```python
from build123d import *

# Parameters (mm, degrees)
F0_W     = 190
F0_H     = 100
F1_DEPTH = 30
F2_T     = -5
F4_DEPTH = 100
F5_R     = 3


with BuildPart() as f1:
    # F0 (on Top) → F1 (new body)
    with BuildSketch(Plane.XY):
        Rectangle(F0_W, F0_H)
    extrude(amount=F1_DEPTH)

    # F2
    f2_openings = [f1.faces().sort_by_distance(p)[0] for p in [
        (0, 0, 30),
    ]]
    offset(amount=F2_T, openings=f2_openings)

    # F3 (on face) → F4 (cut, through all)
    with BuildSketch(Plane.XZ.offset(50)):
        with BuildLine():
            ThreePointArc((-5.1e-08, 5), (8.8388347468, 8.6611652172), (12.5, 17.5))
            Line((12.5, 17.5), (-12.5, 17.5))
            ThreePointArc((-12.5, 17.5), (-8.8388347828, 8.6611652532), (-5.1e-08, 5))
        make_face()
        with BuildLine():
            ThreePointArc((-12.5, 17.5), (-8.8388347699, 26.3388347597), (-1.44e-08, 30))
            Line((-1.44e-08, 30), (-12.5, 30))
            Line((-12.5, 30), (-12.5, 17.5))
        make_face()
        with BuildLine():
            Line((-12.5, 17.5), (12.5, 17.5))
            ThreePointArc((12.5, 17.5), (8.8388347597, 26.3388347699), (-1.44e-08, 30))
            ThreePointArc((-1.44e-08, 30), (-8.8388347699, 26.3388347597), (-12.5, 17.5))
        make_face()
        with BuildLine():
            ThreePointArc((-1.44e-08, 30), (8.8388347597, 26.3388347699), (12.5, 17.5))
            Line((12.5, 17.5), (12.5, 30))
            Line((12.5, 30), (-1.44e-08, 30))
        make_face()
    extrude(amount=-F4_DEPTH, mode=Mode.SUBTRACT)

    # F5
    f5_edges = [f1.edges().sort_by_distance(p)[0] for p in [
        (-12.5, -47.5, 30),
        (12.5, -47.5, 30),
        (-12.5, 47.5, 30),
        (12.5, 47.5, 30),
    ]]
    fillet(f5_edges, radius=F5_R)


solid = f1.part
```
The listing builds one solid part. Answer for the finished solid, in the listing's coordinates (mm). A direction names the side the tool comes from. Give positions to 0.01 mm unless a question says otherwise; leave off trailing zeros. Order: outer loops, then holes, each group sorted by start corner. A loop starts at its lowest first (then second) coordinate and runs counter-clockwise, first axis right, second up.
Item 1: The part is cut by section B-B, the plane y = 41.5. Give the vertices of the cut face in (x, z).
From the geometry:
outline: (-95, 0) - (95, 0) - (95, 30) - (90, 30) - (90, 5) - (-90, 5) - (-90, 30) - (-95, 30) - close
Item 2: For a pull along Y with two mould halves and no side action, classify faces 1 (the face through (90, -1, 17)), 2 (the face through (-1, 1, 5)), 3 (the face through (-91, 0, 30)), 4 (the face through (-1.3, 50, 4.8)) as pulls with the +Y half, pulls with the -Y half, needs draft (parallel to the pull), parting line crosses it, or undercut.
From the geometry:
face 1: undercut
face 2: undercut
face 3: needs draft
face 4: pulls with the +Y half
Item 3: Find the intervals of material crossed by probe 1 along X at (y, z) = (-13, 5.5); probe 2 along Y at (x, z) = (30, 11.5); probe 3 along Z at (x, y) = (56, -18), in increasing order.
From the geometry:
probe 1: x = -95 to -90, 90 to 95
probe 2: y = -50 to -45, 45 to 50
probe 3: z = 0 to 5
Item 4: The part is cut by section A-A, the plane z = 7.5. Give the vertices of the cut face in (x, y), and give its area (3 significant figures).
From the geometry:
outline: (-95, -50) - (-7.5, -50) - (-7.5, -45) - (-90, -45) - (-90, 45) - (-7.5, 45) - (-7.5, 50) - (-95, 50) - close; (7.5, -50) - (95, -50) - (95, 50) - (7.5, 50) - (7.5, 45) - (90, 45) - (90, -45) - (7.5, -45) - close
area: 2,650 mm2
Item 5: The part is cut by section C-C, the plane x = 30. Give the vertices of the cut face in (y, z).
From the geometry:
outline: (-50, 0) - (50, 0) - (50, 30) - (45, 30) - (45, 5) - (-45, 5) - (-45, 30) - (-50, 30) - close
Item 6: Which of the six approach directions +Z, -Z, +X, -X, +Y, -Y give full straight-line access (tool end or side, diameter ignored) to faces 5 (the face through (12.5, -48, 22)), 6 (the face through (-46, 45, 17)), 7 (the face through (-95, -1, 15))?
From the geometry:
face 5: +Z, +Y, -Y
face 6: +Z
face 7: +Z, -Z, -X, +Y, -Y
Item 7: Given pin 1 Ø3 at (x, y) = (-49.5, 1) entering from +Z, flat-ended and moving along its own axis, determine where the tip first touches the part or whether it passes through.
From the geometry:
pin 1: stops at z = 5
